```python
from build123d import *

# Parameters (mm, degrees)
SKETCH1_W           = 1000
SKETCH1_H           = 290
BOSS_EXTRUDE1_DEPTH = 30
SKETCH2_R           = 15
SKETCH2_R_2         = 12.5
BOSS_EXTRUDE2_DEPTH = 500
SKETCH3_R           = 15
SKETCH3_R_2         = 12.5
BOSS_EXTRUDE3_DEPTH = 500


with BuildPart() as part:
    # Sketch1 → Boss-Extrude1 (new body)
    with BuildSketch(Plane.XY):
        Rectangle(SKETCH1_W, SKETCH1_H)
    extrude(amount=BOSS_EXTRUDE1_DEPTH)

    # Sketch2 → Boss-Extrude2 (add)
    with BuildSketch(Plane(origin=(500, 0, 0), x_dir=(0, 0, -1), z_dir=(1, 0, 0))):
        with Locations((-15, 160)):
            Circle(SKETCH2_R)
        with Locations((-15, 160)):
            Circle(SKETCH2_R_2, mode=Mode.SUBTRACT)
        with BuildLine():
            ThreePointArc((-15, 145), (-25.606601718, 149.393398282), (-30, 160))
            Line((-30, 160), (-30, 145))
            Line((-30, 145), (-15, 145))
        make_face()
        with BuildLine():
            Line((0, 145), (0, 160))
            ThreePointArc((0, 160), (-4.393398282, 149.393398282), (-15, 145))
            Line((-15, 145), (0, 145))
        make_face()
    extrude(amount=-BOSS_EXTRUDE2_DEPTH)

    # Sketch3 → Boss-Extrude3 (add)
    with BuildSketch(Plane.ZY.offset(500)):
        with BuildLine():
            Line((0, -145), (0, -160))
            ThreePointArc((0, -160), (4.393398282, -149.393398282), (15, -145))
            Line((15, -145), (0, -145))
        make_face()
        with Locations((15, -160)):
            Circle(SKETCH3_R)
        with Locations((15, -160)):
            Circle(SKETCH3_R_2, mode=Mode.SUBTRACT)
        with BuildLine():
            ThreePointArc((15, -145), (25.606601718, -149.393398282), (30, -160))
            Line((30, -160), (30, -145))
            Line((30, -145), (15, -145))
        make_face()
    extrude(amount=-BOSS_EXTRUDE3_DEPTH)


solid = part.part
```
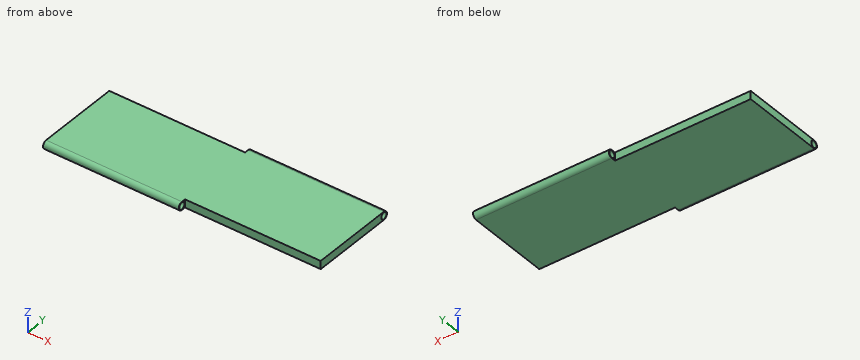
CAD build for the part. Positions are in the model's coordinates, mm. Round coordinates to 2 decimals unless told otherwise and drop trailing zeros. Order: outer loops, then holes, each group sorted by start corner. A loop starts at its lowest first (then second) coordinate and runs counter-clockwise, first axis right, second up.
Q1. Slice it at B-B (x = 147). Write the cut outline in (y, z).
Q2. Slice it at A-A (z = 15). Write the cut outline in (x, y), and give its area (3 significant figures).
Q3. Drop flat-ended pins along their axis: pin 1 (1 mm diameter, centred on x = 343.5, z = 13.5, fed in from -Y); pin 2 (1.5 mm diameter, centred on x = -277.5, y = 124, fed in from -Z). Give the stop position or say it passes through.
Q4. Wall check: L1, parallel to Y at x = -381, z = 15; L2, parallel to Y at x = 122, z = 15; L3, parallel to Y at x = 384.5, z = 28. Give the ranges that are in metal, low to high.
Results below:
1. outline: (-145, 0) - (160, 0) arc R15 ccw to (160, 30) - (-145, 30) - close; hole circle Ø25 at (160, 15)
2. outline: (-500, -175) - (0, -175) - (0, -172.5) - (-500, -172.5) - close; (-500, -147.5) - (0, -147.5) - (0, -145) - (500, -145) - (500, 147.5) - (0, 147.5) - (0, 145) - (-500, 145) - close; (0, 172.5) - (500, 172.5) - (500, 175) - (0, 175) - close
2. area: 295,000 mm2
3. pin 1: stops at y = -145
3. pin 2: stops at z = 0
4. L1: y = -175 to -172.5, -147.5 to 145
4. L2: y = -145 to 147.5, 172.5 to 175
4. L3: y = -145 to 167.48
